from build123d import *

# Parameters (mm, degrees)
SKETCH_1_W           = 200
SKETCH_1_H           = 40
EXTRUDE_1_DEPTH      = 100
SKETCH_1_3_W         = 200
SKETCH_1_3_H         = 40
EXTRUDE_2_DEPTH      = 130
SKETCH_10_W          = 200
SKETCH_10_H          = 40
EXTRUDE_3_DEPTH      = 160
SKETCH_12_R          = 5
CUT_EXTRUDE_8_DEPTH  = 50
CUT_EXTRUDE_8_DRAFT  = -1
SKETCH_12_5_R        = 5
CUT_EXTRUDE_9_DEPTH  = 45
CUT_EXTRUDE_9_DRAFT  = -1
SKETCH_12_6_R        = 5
CUT_EXTRUDE_10_DEPTH = 40
CUT_EXTRUDE_10_DRAFT = -1
SKETCH_12_7_R        = 5
CUT_EXTRUDE_11_DEPTH = 35
CUT_EXTRUDE_11_DRAFT = -1
SKETCH_12_8_R        = 5
CUT_EXTRUDE_12_DEPTH = 30
CUT_EXTRUDE_12_DRAFT = -1


with BuildPart() as part:
    # Эскиз1 → Бобышка-Вытянуть1 (new body)
    with BuildSketch(Plane.XY):
        with Locations((100, 20)):
            Rectangle(SKETCH_1_W, SKETCH_1_H)
    extrude(amount=EXTRUDE_1_DEPTH)

    # Эскиз1<3> → Бобышка-Вытянуть2 (add)
    with BuildSketch(Plane.XY):
        with Locations((100, 60)):
            Rectangle(SKETCH_1_3_W, SKETCH_1_3_H)
    extrude(amount=EXTRUDE_2_DEPTH)

    # Эскиз10 → Бобышка-Вытянуть3 (add)
    with BuildSketch(Plane(origin=(0, 0, 0), x_dir=(-1, 0, 0), z_dir=(0, 0, -1))):
        with Locations((-100, 100)):
            Rectangle(SKETCH_10_W, SKETCH_10_H)
    extrude(amount=-EXTRUDE_3_DEPTH)


with BuildPart() as cut_extrude_8_tool:
    # Эскиз12 → Вырез-Вытянуть8 (with draft: the straight prism first)
    with BuildSketch(Plane.XY.offset(130)):
        with Locations((24.220497744, 60)):
            Circle(SKETCH_12_R)
    extrude(amount=-CUT_EXTRUDE_8_DEPTH)
    # Вырез-Вытянуть8: the draft: its side faces are tilted about the plane it starts from
    cut_extrude_8_sides = [cut_extrude_8_tool.faces().sort_by_distance(p)[0] for p in [
        (19.220497744, 60, 105),
    ]]
    draft(cut_extrude_8_sides, Plane.XY.offset(130), CUT_EXTRUDE_8_DRAFT)


with BuildPart() as part_1:
    add(part.part)

    # Вырез-Вытянуть8: cut by cut_extrude_8_tool
    add(cut_extrude_8_tool.part, mode=Mode.SUBTRACT)


with BuildPart() as cut_extrude_9_tool:
    # Эскиз12<5> → Вырез-Вытянуть9 (with draft: the straight prism first)
    with BuildSketch(Plane.XY.offset(130)):
        with Locations((60.740492413, 60)):
            Circle(SKETCH_12_5_R)
    extrude(amount=-CUT_EXTRUDE_9_DEPTH)
    # Вырез-Вытянуть9: the draft: its side faces are tilted about the plane it starts from
    cut_extrude_9_sides = [cut_extrude_9_tool.faces().sort_by_distance(p)[0] for p in [
        (55.740492413, 60, 107.5),
    ]]
    draft(cut_extrude_9_sides, Plane.XY.offset(130), CUT_EXTRUDE_9_DRAFT)


with BuildPart() as part_2:
    add(part_1.part)

    # Вырез-Вытянуть9: cut by cut_extrude_9_tool
    add(cut_extrude_9_tool.part, mode=Mode.SUBTRACT)


with BuildPart() as cut_extrude_10_tool:
    # Эскиз12<6> → Вырез-Вытянуть10 (with draft: the straight prism first)
    with BuildSketch(Plane.XY.offset(130)):
        with Locations((100, 60)):
            Circle(SKETCH_12_6_R)
    extrude(amount=-CUT_EXTRUDE_10_DEPTH)
    # Вырез-Вытянуть10: the draft: its side faces are tilted about the plane it starts from
    cut_extrude_10_sides = [cut_extrude_10_tool.faces().sort_by_distance(p)[0] for p in [
        (95, 60, 110),
    ]]
    draft(cut_extrude_10_sides, Plane.XY.offset(130), CUT_EXTRUDE_10_DRAFT)


with BuildPart() as part_3:
    add(part_2.part)

    # Вырез-Вытянуть10: cut by cut_extrude_10_tool
    add(cut_extrude_10_tool.part, mode=Mode.SUBTRACT)


with BuildPart() as cut_extrude_11_tool:
    # Эскиз12<7> → Вырез-Вытянуть11 (with draft: the straight prism first)
    with BuildSketch(Plane.XY.offset(130)):
        with Locations((137.238261218, 60)):
            Circle(SKETCH_12_7_R)
    extrude(amount=-CUT_EXTRUDE_11_DEPTH)
    # Вырез-Вытянуть11: the draft: its side faces are tilted about the plane it starts from
    cut_extrude_11_sides = [cut_extrude_11_tool.faces().sort_by_distance(p)[0] for p in [
        (132.238261218, 60, 112.5),
    ]]
    draft(cut_extrude_11_sides, Plane.XY.offset(130), CUT_EXTRUDE_11_DRAFT)


with BuildPart() as part_4:
    add(part_3.part)

    # Вырез-Вытянуть11: cut by cut_extrude_11_tool
    add(cut_extrude_11_tool.part, mode=Mode.SUBTRACT)


with BuildPart() as cut_extrude_12_tool:
    # Эскиз12<8> → Вырез-Вытянуть12 (with draft: the straight prism first)
    with BuildSketch(Plane.XY.offset(130)):
        with Locations((173.42575674, 60)):
            Circle(SKETCH_12_8_R)
    extrude(amount=-CUT_EXTRUDE_12_DEPTH)
    # Вырез-Вытянуть12: the draft: its side faces are tilted about the plane it starts from
    cut_extrude_12_sides = [cut_extrude_12_tool.faces().sort_by_distance(p)[0] for p in [
        (168.42575674, 60, 115),
    ]]
    draft(cut_extrude_12_sides, Plane.XY.offset(130), CUT_EXTRUDE_12_DRAFT)


with BuildPart() as part_5:
    add(part_4.part)

    # Вырез-Вытянуть12: cut by cut_extrude_12_tool
    add(cut_extrude_12_tool.part, mode=Mode.SUBTRACT)


solid = part_5.part
Check sheet for the modelled part. Datum: model origin and axes. Units: mm. A direction names the side the tool comes from. Give positions to 0.01 mm unless a question says otherwise; leave off trailing zeros. Write each loop counter-clockwise with the first axis right and the second up, starting at its lowest first coordinate (ties: lowest second). Pieces come first, ordered by that corner, then holes. Notation, with made-up numbers: (74, 43.25) -> (104, 43.25) arc R22 ccw to (104, 49.25) -> close; hole circle Ø5 at (33, -18.5). An arc over 180 degrees is marked (long way). Use one line per item in the form item = value. Start each with the question number.
1. Section check C-C (y = 74.5). Record the cut outline in (x, z), and give its area (3 significant figures).
2. Mould release check, pull along X, two halves, no side actions. Record for faces 1 (the flat face through (99, 40, 115)), 2 (the flat face through (137, 60, 95)), 3 (the flat face through (0, 59, 61)): pulls with the +X half, pulls with the -X half, needs draft (parallel to the pull), parting line crosses it, or undercut.
3. Section check A-A (x = 37.5). Record the cut outline in (y, z).
4. Go/stop test with flat-tipped pins: P1, Ø7, axis at x = 172.5, y = 60, coming from the +Z side; P2, Ø4.5, axis at x = 137, y = 59, coming from the +Z side; P3, Ø9, axis at x = 118, z = 114.5, coming from the -Y side; P4, Ø2, axis at x = 64, y = 74, coming from the -Z side. Record where each tip stops, or that it passes through.
5. Access from +Z, -Z, +X, -X, +Y, -Y to the whole of each face (thin tool, end or side, straight path). Record for faces 4 (the conical face through (132.544, 60.207, 112.745)), 5 (the flat face through (99, 51, 130)), 6 (the flat face through (99, 0, 49)).
6. Thickness scan on line 1 along Y through (x, z) = (110.5, 120.5); line 2 along Z through (x, y) = (115.5, 55.5); line 3 along Z through (x, y) = (90.5, 7). Record the ranges inside material, lowest first. Write a range as from..to.
7. Section check B-B (z = 122). Record the cut outline in (x, y).
8. Section check D-D (y = 21.5). Record the cut outline in (x, z), and give its area (3 significant figures).
Conclusion:
q1.outline = (0, 0) -> (200, 0) -> (200, 130) -> (0, 130) -> close
q1.area = 26,000 mm²
q2.face_1 = needs draft
q2.face_2 = undercut
q2.face_3 = pulls with the -X half
q3.outline = (0, 0) -> (120, 0) -> (120, 160) -> (80, 160) -> (80, 130) -> (40, 130) -> (40, 100) -> (0, 100) -> close
q4.P1 = 100
q4.P2 = 95
q4.P3 = 40
q4.P4 = 0
q5.face_4 = +Z
q5.face_5 = +Z, +X, -X, -Y
q5.face_6 = +Z, -Z, +X, -X, -Y
q6.line_1 = 40..120
q6.line_2 = 0..130
q6.line_3 = 0..100
q7.outline = (0, 40) -> (200, 40) -> (200, 120) -> (0, 120) -> close; hole circle Ø9.72 at (24.22, 60); hole circle Ø9.72 at (60.74, 60); hole circle Ø9.72 at (100, 60); hole circle Ø9.72 at (137.24, 60); hole circle Ø9.72 at (173.43, 60)
q8.outline = (0, 0) -> (200, 0) -> (200, 100) -> (0, 100) -> close
q8.area = 20,000 mm²
